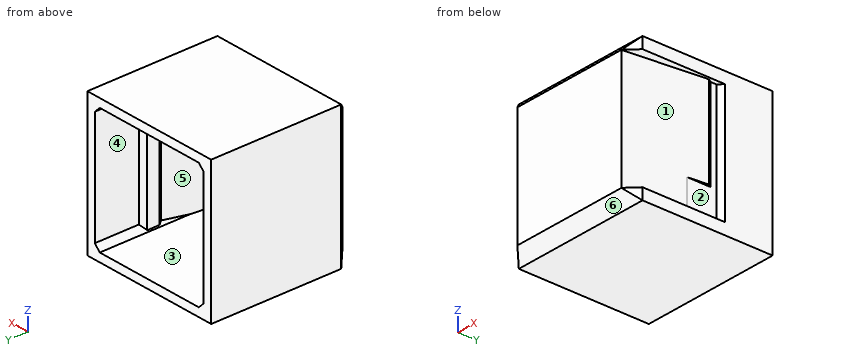
from build123d import *

# Parameters (mm, degrees)
SKIZZE1_W                       = 25
SKIZZE1_H                       = 25
AUFSATZ_LINEAR_AUSTRAGEN1_DEPTH = 25
FASE1_SIZE                      = 2
SCHNITT_LINEAR_START            = -2
SCHNITT_LINEAR_AUSTRAGEN1_DEPTH = 21
WANDUNG1_START                  = -11
WANDUNG1_DEPTH                  = 22
WANDUNG1_START_2                = -12
WANDUNG1_2_DEPTH                = 22
FASE2_SIZE                      = 1
SCHNITT_LINEAR_AUSTRAGEN2_DEPTH = 5


with BuildPart() as part:
    # Skizze1 → Aufsatz-Linear austragen1 (new body)
    with BuildSketch(Plane(origin=(0, 0, 0), x_dir=(1, 0, 0), z_dir=(0, 1, 0))):
        Rectangle(SKIZZE1_W, SKIZZE1_H)
    extrude(amount=AUFSATZ_LINEAR_AUSTRAGEN1_DEPTH)

    # Fase1
    fase1_edges = [part.edges().sort_by_distance(p)[0] for p in [
        (0, 0, 12.5),
        (-12.5, 0, 0),
        (0, 0, -12.5),
        (12.5, 0, 0),
    ]]
    chamfer(fase1_edges, length=FASE1_SIZE)

    # Skizze3 → Schnitt-Linear austragen1 (cut)
    with BuildSketch(Plane.XY.offset(12.5).offset(SCHNITT_LINEAR_START)):
        Polygon((11.691418824, 15.798054248), (11.691418824, 14.698054248), (12.085432918, 14.119124044), (10.5, 0), (12.5, 0), (12.5, 16.576443976), align=None)
    extrude(amount=-SCHNITT_LINEAR_AUSTRAGEN1_DEPTH, mode=Mode.SUBTRACT)

    # Wandung1: read off the stored shape, not the designer's step
    # Wandung1 outline → Wandung1 (cut)
    with BuildSketch(Plane.XY.offset(WANDUNG1_START)):
        Polygon((10.191418824, 14.236037823), (10.191418824, 16.4361557), (11, 17.214545429), (11, 25), (-11, 25), (-11, 2.621320344), (-9.878679656, 1.5), (9.159007508, 1.5), (10.532808529, 13.734429342), align=None)
    extrude(amount=WANDUNG1_DEPTH, mode=Mode.SUBTRACT)

    # Wandung1 2 outline → Wandung1 2 (add)
    with BuildSketch(Plane.YZ.offset(WANDUNG1_START_2)):
        Polygon((2.621320344, -11), (1.5, -9.878679656), (1.5, -11), align=None)
        Polygon((1.5, 9.878679656), (2.621320344, 11), (1.5, 11), align=None)
    extrude(amount=WANDUNG1_2_DEPTH)

    # Fase2
    fase2_edges = [part.edges().sort_by_distance(p)[0] for p in [
        (11, 21.107272714, 11),
        (-11, 13.810660172, 11),
        (-11, 13.810660172, -11),
        (11, 21.107272714, -11),
    ]]
    chamfer(fase2_edges, length=FASE2_SIZE)

    # Skizze4 → Schnitt-Linear austragen2 (cut)
    with BuildSketch(Plane.XY.offset(-10.5)):
        Polygon((11.691418824, 15.798054248), (11.691418824, 11.720195976), (11.691418824, 10.610218801), (10.5, 0), (12.5, 2), (12.5, 16.576443976), align=None)
    extrude(amount=SCHNITT_LINEAR_AUSTRAGEN2_DEPTH, mode=Mode.SUBTRACT)


solid = part.part
Verification items for the finished model (mm, model axes). Face numbers are marked on the shaded views. A direction names the side the tool comes from. Coordinates: 2 decimals unless noted, no trailing zeros. Write each loop counter-clockwise with the first axis right and the second up, starting at its lowest first coordinate (ties: lowest second). Pieces come first, ordered by that corner, then holes. Notation, with made-up numbers: M -28.5,-26.75 L 27.5,-26.75 A18 cw 27.5,-18.75 Z; hole C 71,74 d10. An arc over 180 degrees is marked long. Use CSV: the item, a comma, the result in double quotes.
Q1. Mould release check, pull along Y, two halves, no side actions. Record for the marked faces 4, 5 and 6: pulls with the +Y half, pulls with the -Y half, needs draft (parallel to the pull), parting line crosses it, or undercut.
Computed values:
face 4,"needs draft"
face 5,"undercut"
face 6,"pulls with the -Y half"
Q2. Thickness scan on line 1 along Z through (x, y) = (-8.5, 15.5); line 2 along X through (y, z) = (15, -9.25). Record the ranges inside material, lowest first. Write a range as [from, to].
Computed values:
line 1,"[-12.5, -11], [11, 12.5]"
line 2,"[-12.5, -11], [10.19, 11.69]"
Q3. Set-up check for the marked faces 1, 2 and 3: record each of +Z, -Z, +X, -X, +Y, -Y from which the full face is reachable in a straight line by a thin tool's end or side.
Computed values:
face 1,"+X, -Y"
face 2,"+X"
face 3,"+Y"
Q4. Section check D-D, the plane y = 12.5. Enter the section's corners in (x, z), and give its area (3 significant figures).
Computed values:
outline,"M -12.5,-12.5 L 12.5,-12.5 L 12.5,-10.5 L 11.69,-10.5 L 11.69,-5.5 L 11.9,-5.5 L 11.9,10.5 L 12.5,10.5 L 12.5,12.5 L -12.5,12.5 Z; hole M -11,-10 L -10,-11 L 10,-11 L 10.39,-10.61 L 10.39,10.61 L 10,11 L -10,11 L -11,10 Z"
area,"142 mm²"
Q5. Go/stop test with flat-tipped pins: P1, Ø1, axis at x = 4.5, z = -5.5, coming from the -Y side; P2, Ø5.5, axis at x = 1.5, z = -4, coming from the +Y side; P3, Ø5.5, axis at y = 12, z = -2.5, coming from the +X side. Record where each tip stops, or that it passes through.
Computed values:
P1,"y = 0"
P2,"y = 1.5"
P3,"x = 12.09"
Q6. Section check A-A, the plane y = 19.5. Enter the section's corners in (x, z).
Computed values:
outline,"M -12.5,-12.5 L 12.5,-12.5 L 12.5,12.5 L -12.5,12.5 Z; hole M -11,-10 L -10,-11 L 10,-11 L 11,-10 L 11,10 L 10,11 L -10,11 L -11,10 Z"
Q7. Section check B-B, the plane x = 5.25. Enter the section's corners in (y, z), and give its area (3 significant figures).
Computed values:
outline,"M 0,-10.5 L 2,-12.5 L 25,-12.5 L 25,-11 L 2.62,-11 L 1.5,-9.88 L 1.5,9.88 L 2.62,11 L 25,11 L 25,12.5 L 2,12.5 L 0,10.5 Z"
area,"105 mm²"
Q8. Section check C-C, the plane z = -5. Enter the section's corners in (x, y), and give its area (3 significant figures).
Computed values:
outline,"M -12.5,2 L -10.5,0 L 10.5,0 L 12.09,14.12 L 11.69,14.7 L 11.69,15.8 L 12.5,16.58 L 12.5,25 L 11,25 L 11,17.21 L 10.19,16.44 L 10.19,14.24 L 10.53,13.73 L 9.16,1.5 L -9.88,1.5 L -11,2.62 L -11,25 L -12.5,25 Z"
area,"105 mm²"
